from build123d import *

# Parameters (mm, degrees)
SKETCH1_W           = 151
SKETCH1_H           = 118
SKETCH1_W_2         = 148
SKETCH1_H_2         = 115
BOSS_EXTRUDE1_DEPTH = 5
SKETCH2_W           = 151
SKETCH2_H           = 118
SKETCH2_W_2         = 132
SKETCH2_H_2         = 102
BOSS_EXTRUDE2_DEPTH = 1.5


with BuildPart() as part:
    # Sketch1 → Boss-Extrude1 (new body)
    with BuildSketch(Plane(origin=(0, 0, 0), x_dir=(1, 0, 0), z_dir=(0, 1, 0))):
        Rectangle(SKETCH1_W, SKETCH1_H)
        Rectangle(SKETCH1_W_2, SKETCH1_H_2, mode=Mode.SUBTRACT)
    extrude(amount=BOSS_EXTRUDE1_DEPTH)

    # Sketch2 → Boss-Extrude2 (add)
    with BuildSketch(Plane(origin=(0, 5, 0), x_dir=(1, 0, 0), z_dir=(0, 1, 0))):
        Rectangle(SKETCH2_W, SKETCH2_H)
        with Locations((0, 1.5)):
            Rectangle(SKETCH2_W_2, SKETCH2_H_2, mode=Mode.SUBTRACT)
    extrude(amount=BOSS_EXTRUDE2_DEPTH)


solid = part.part
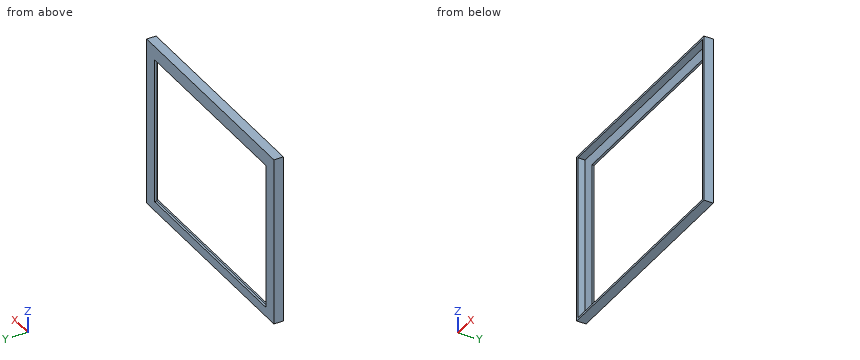
Check sheet for the modelled part. Datum: model origin and axes. Units: mm. Round coordinates to 2 decimals unless told otherwise and drop trailing zeros. Write each loop counter-clockwise with the first axis right and the second up, starting at its lowest first coordinate (ties: lowest second). Pieces come first, ordered by that corner, then holes. Notation, with made-up numbers: (51.25, -34) - (105.25, -34) arc R24 cw to (105.25, -23) - close; hole circle Ø2 at (-20, 88). An arc over 180 degrees is marked (long way). Return JSON: item names as keys, results as strings.
Q1. Cross-section at A-A (x = 19). Record the boundary of the cut face in (y, z).
Returned:
{"outline": "(0, -59) - (6.5, -59) - (6.5, -52.5) - (5, -52.5) - (5, -57.5) - (0, -57.5) - close; (0, 57.5) - (5, 57.5) - (5, 49.5) - (6.5, 49.5) - (6.5, 59) - (0, 59) - close"}
Q2. Scan lines: L1, parallel to Z at x = 37, y = 5.25; L2, parallel to Z at x = 34.5, y = 2; L3, parallel to X at y = 3, z = 16.5. Record each from-to range of solid material in increasing order. Write a range as from..to.
Returned:
{"L1": "z = -59..-52.5, 49.5..59", "L2": "z = -59..-57.5, 57.5..59", "L3": "x = -75.5..-74, 74..75.5"}
Q3. Cross-section at C-C (z = -16.5). Record the boundary of the cut face in (x, y), then the cut area to 3 significant figures.
Returned:
{"outline": "(-75.5, 0) - (-74, 0) - (-74, 5) - (-66, 5) - (-66, 6.5) - (-75.5, 6.5) - close; (66, 5) - (74, 5) - (74, 0) - (75.5, 0) - (75.5, 6.5) - (66, 6.5) - close", "area": "43.5 mm²"}
Q4. Cross-section at B-B (y = 2). Record the boundary of the cut face in (x, z).
Returned:
{"outline": "(-75.5, -59) - (75.5, -59) - (75.5, 59) - (-75.5, 59) - close; hole (-74, -57.5) - (74, -57.5) - (74, 57.5) - (-74, 57.5) - close"}
